Can you work these out from the model? Positions are in its coordinate system, mm. Round coordinates to 2 decimals unless told otherwise and drop trailing zeros. Loops run counter-clockwise (first coordinate to the right, second up) from the corner with the lowest first, then second, coordinate; pieces in that order, holes last.
from build123d import *

# Parameters (mm, degrees)
BOX018_W        = 27
BOX018_H        = 44
BOX018_DEPTH    = 5
BOX019_W        = 80
BOX019_H        = 44
BOX019_DEPTH    = 5
CHAMFER016_SIZE = 25
FILLET004003_R  = 3


with BuildPart() as cube018:
    # Box018 → Box018 (new body)
    with BuildSketch(Plane(origin=(-27, -44, -5), x_dir=(1, 0, 0), z_dir=(0, 0, 1))):
        with Locations((13.5, 22)):
            Rectangle(BOX018_W, BOX018_H)
    extrude(amount=BOX018_DEPTH)


with BuildPart() as fillet004003:
    # Box019 → Box019 (new body)
    with BuildSketch(Plane(origin=(0, -14, -5), x_dir=(1, 0, 0), z_dir=(0, 0, 1))):
        with Locations((40, 22)):
            Rectangle(BOX019_W, BOX019_H)
    extrude(amount=BOX019_DEPTH)

    # Fusion006002011004053036004001003009006003: union Cube018
    add(cube018.part)

    # Chamfer016
    chamfer016_edges = [fillet004003.edges().sort_by_distance(p)[0] for p in [
        (0, -14, -2.5),
    ]]
    chamfer(chamfer016_edges, length=CHAMFER016_SIZE)

    # Fillet004003
    fillet004003_edges = [fillet004003.edges().sort_by_distance(p)[0] for p in [
        (80, -14, -2.5),
        (80, 30, -2.5),
        (0, 30, -2.5),
        (0, -44, -2.5),
        (-27, -44, -2.5),
        (-27, 0, -2.5),
    ]]
    fillet(fillet004003_edges, radius=FILLET004003_R)


solid = fillet004003.part
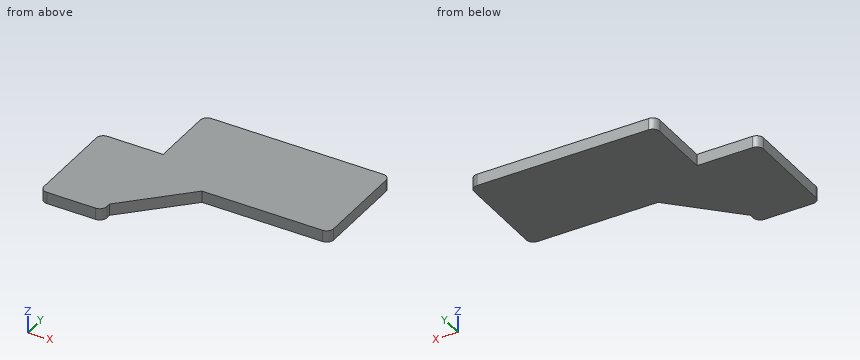
(1) If we section it at B-B, the plane x = 4.5: List the corners of the cut face in (y, z) for me.
Worked answers:
outline: (-34.5, -5) - (30, -5) - (30, 0) - (-34.5, 0) - close
(2) Will these pins go through, and if not, where does the flat tip stop? P1, Ø6, axis at x = 13, y = 7, coming from the +Z side; P2, Ø3, axis at y = 21.5, z = -0.5, coming from the -X side.
Worked answers:
P1: stops at z = 0
P2: stops at x = 0
(3) If I drill on line 1 (Y direction, x = 72.5, z = -4.3); line 2 (X direction, y = 9.5, z = -1.1); line 3 (Y direction, x = -4.5, z = -0.4), over which ranges is the centre line in solid material (lowest first)?
Worked answers:
line 1: y = -14 to 30
line 2: x = 0 to 80
line 3: y = -44 to 0
(4) If we section it at A-A, the plane z = -3.4: List the corners of the cut face in (x, y) for me.
Worked answers:
outline: (-27, -41) arc R3 ccw to (-24, -44) - (-3, -44) arc R3 ccw to (0, -41) - (0, -39) - (25, -14) - (77, -14) arc R3 ccw to (80, -11) - (80, 27) arc R3 ccw to (77, 30) - (3, 30) arc R3 ccw to (0, 27) - (0, 0) - (-24, 0) arc R3 ccw to (-27, -3) - close
(5) If we section it at C-C, the plane y = -37: List the corners of the cut face in (x, z) for me.
Worked answers:
outline: (-27, -5) - (2, -5) - (2, 0) - (-27, 0) - close
